```python
from build123d import *

# Parameters (mm, degrees)
P_IDAT_VYSUNUT_M1_DEPTH = 6


with BuildPart() as part:
    # Skica1 → Přidat vysunutím1 (new body)
    with BuildSketch(Plane.XY):
        with BuildLine():
            ThreePointArc((54.607141883, 21.260763283), (0, -58.6), (-54.607141883, 21.260763283))
            ThreePointArc((-54.607141883, 21.260763283), (0, 58.6), (54.607141883, 21.260763283))
        make_face()
        with BuildLine():
            ThreePointArc((-46.248555772, -14.934225425), (0, -48.6), (46.248555772, -14.934225425))
            ThreePointArc((46.248555772, -14.934225425), (54.72152315, 0.001816211), (46.247564334, 14.937295377))
            ThreePointArc((46.247564334, 14.937295377), (0, 48.6), (-46.247564334, 14.937295377))
            ThreePointArc((-46.247564334, 14.937295377), (-54.72152315, 0.001816211), (-46.248555772, -14.934225425))
        make_face(mode=Mode.SUBTRACT)
    extrude(amount=P_IDAT_VYSUNUT_M1_DEPTH)


solid = part.part
```
Input: part model. Units: mm. Frame: model coordinates. A direction names the side the tool comes from. Coordinates: 2 decimals unless noted, no trailing zeros. Loops run counter-clockwise (first coordinate to the right, second up) from the corner with the lowest first, then second, coordinate; pieces in that order, holes last. Notation, with made-up numbers: M 71,70 L 96,70 A15 cw 96,74 Z; hole C -12,79.5 d8. An arc over 180 degrees is marked long. Answer in a Markdown table with one row per item.
1. First-contact query: pin 1 (1.5 mm diameter, centred on x = -39.5, z = 1.5, fed in from -Y); pin 2 (1.5 mm diameter, centred on y = 23.5, z = 2, fed in from -X); pin 3 (1 mm diameter, centred on y = 9.5, z = 3, fed in from +X). Flat tips, straight axial feed; report the tip coordinate or a pass-through.
Response:
| item | result |
|---|---|
| pin 1 | stops at y = -43.96 |
| pin 2 | stops at x = -54 |
| pin 3 | stops at x = 57.9 |
2. Reachability of faces 3 (the flat face through (9, 48, 0)), 4 (the cylindrical face through (-54.72, 0.25, 2.96)) from +Z, -Z, +X, -X, +Y, -Y: full face, straight path, thin tool, end or side. Return the list, or none.
Response:
| item | result |
|---|---|
| face 3 | -Z, +X, -X, +Y, -Y |
| face 4 | +Z, -Z |
3. Material intervals for line 1 (Y direction, x = -1.5, z = 0.5); line 2 (Y direction, x = -8, z = 5.6); line 3 (X direction, y = 25, z = 3.15), sorted ascending.
Response:
| item | result |
|---|---|
| line 1 | y = -58.58 to -48.58, 48.58 to 58.58 |
| line 2 | y = -58.05 to -47.94, 47.94 to 58.05 |
| line 3 | x = -53 to -41.68, 41.68 to 53 |
4. Section A-A, the plane x = 0. Output: boundary loops of the cut face in (y, z), then the cut area to 3 significant figures.
Response:
| item | result |
|---|---|
| outline | M -58.6,0 L -48.6,0 L -48.6,6 L -58.6,6 Z; M 48.6,0 L 58.6,0 L 58.6,6 L 48.6,6 Z |
| area | 120 mm2 |
5. Section B-B, the plane y = 0. Output: boundary loops of the cut face in (x, z).
Response:
| item | result |
|---|---|
| outline | M -58.6,0 L -54.72,0 L -54.72,6 L -58.6,6 Z; M 54.72,0 L 58.6,0 L 58.6,6 L 54.72,6 Z |
6. Section C-C, the plane z = 2. Output: boundary loops of the cut face in (x, y).
Response:
| item | result |
|---|---|
| outline | C 0,0 d117.2; hole M -46.25,-14.93 A48.6 ccw 46.25,-14.93 A17.4 ccw 46.25,14.94 A48.6 ccw -46.25,14.94 A17.4 ccw Z |
7. Draft query along X for faces 1 (the flat face through (9, 48, 6)), 2 (the cylindrical face through (54.72, -0.25, 2.96)). Return one class per face: pulls with the +X half, pulls with the -X half, needs draft (parallel to the pull), parting line crosses it, or undercut.
Response:
| item | result |
|---|---|
| face 1 | needs draft |
| face 2 | undercut |
